from build123d import *

# Parameters (mm, degrees)
SKETCH_1_W          = 200
SKETCH_1_H          = 170
EXTRUDE_1_DEPTH     = 1
SKETCH_2_R          = 52.5
CUT_EXTRUDE_1_DEPTH = 2
SKETCH_3_R          = 1.6
CUT_EXTRUDE_2_DEPTH = 1
SKETCH_6_W          = 1.1
SKETCH_6_H          = 170
CUT_EXTRUDE_4_DEPTH = 10
FILLET_1_R          = 2
SKETCH_8_R          = 1.6
CUT_EXTRUDE_5_DEPTH = 10


with BuildPart() as part:
    # 草图1 → 凸台-拉伸1 (new body)
    with BuildSketch(Plane.XY):
        Rectangle(SKETCH_1_W, SKETCH_1_H)
    extrude(amount=EXTRUDE_1_DEPTH)

    # 草图2 → 切除-拉伸1 (cut)
    with BuildSketch(Plane(origin=(0, 0, 0), x_dir=(-1, 0, 0), z_dir=(0, 0, -1))):
        with Locations((0, -95)):
            Circle(SKETCH_2_R)
    extrude(amount=-CUT_EXTRUDE_1_DEPTH, mode=Mode.SUBTRACT)

    # 草图3 → 切除-拉伸2 (cut)
    with BuildSketch(Plane(origin=(0, 0, 0), x_dir=(-1, 0, 0), z_dir=(0, 0, -1))):
        with Locations((95, 14.722484501)):
            Circle(SKETCH_3_R)
        with Locations((95, -5.277515499)):
            Circle(SKETCH_3_R)
    cut_extrude_2 = extrude(amount=-CUT_EXTRUDE_2_DEPTH, mode=Mode.SUBTRACT)

    # 镜向1: 切除-拉伸2 across plane
    add(cut_extrude_2.mirror(Plane(origin=(0, 0, 0), x_dir=(0, 0, 1), z_dir=(1, 0, 0))), mode=Mode.SUBTRACT)

    # 草图6 → 切除-拉伸4 (cut)
    with BuildSketch(Plane(origin=(0, 0, 0), x_dir=(-1, 0, 0), z_dir=(0, 0, -1))):
        with Locations((-99.45, 0)):
            Rectangle(SKETCH_6_W, SKETCH_6_H)
    extrude(amount=-CUT_EXTRUDE_4_DEPTH, mode=Mode.SUBTRACT)

    # 圆角1
    fillet_1_edges = [part.edges().sort_by_distance(p)[0] for p in [
        (51.53882032, -85, 0.5),
        (-51.53882032, -85, 0.5),
        (98.9, 85, 0.5),
        (98.9, -85, 0.5),
        (-100, -85, 0.5),
        (-100, 85, 0.5),
    ]]
    fillet(fillet_1_edges, radius=FILLET_1_R)

    # 草图8 → 切除-拉伸5 (cut)
    with BuildSketch(Plane(origin=(0, 0, 0), x_dir=(-1, 0, 0), z_dir=(0, 0, -1))):
        with Locations((-92.1, 44.5)):
            Circle(SKETCH_8_R)
        with Locations((-92.1, 30.5)):
            Circle(SKETCH_8_R)
        with Locations((-92.1, -30.5)):
            Circle(SKETCH_8_R)
        with Locations((-92.1, -44.5)):
            Circle(SKETCH_8_R)
    extrude(amount=-CUT_EXTRUDE_5_DEPTH, mode=Mode.SUBTRACT)


solid = part.part
Source: CAD feature listing. Evaluate the final solid. Frame: model axes, mm. Round coordinates to 2 decimals unless told otherwise and drop trailing zeros. Loops run counter-clockwise (first coordinate to the right, second up) from the corner with the lowest first, then second, coordinate; pieces in that order, holes last. Notation, with made-up numbers: (-3, 7.25) - (38, 7.25) arc R11 cw to (38, 21.25) - close; hole circle Ø9 at (-4.5, 2.5). An arc over 180 degrees is marked (long way). Write item = value, one per line. Start each with the question number.
(1) Pull-direction query (X, two-part tool) for faces 1 (the face through (-2, 1, 0)), 2 (the face through (-0.99, -42.51, 0.49)); classes: +X half, -X half, draft (parallel to the pull), parting line (faces both ways), or undercut.
(2) Pin query (flat end, axial travel): pin 1 (1 mm diameter, centred on x = 76, y = -57.5, fed in from -Z). Return the tip coordinate at first contact, or that it passes through.
(3) Section query B-B, the plane z = 0.45. State how many separate pieces and enclosed holes the cut face has, plus the area to 3 significant figures.
(4) Section query A-A, the plane y = -55.5. Output: boundary loops of the cut face in (x, z).
(5) Ray query, line 1 along Y through (x, z) = (95, 0.6); line 2 along Y through (x, z) = (92.1, 0.35); line 3 along Y through (x, z) = (21.5, 0.8). Return the intervals inside material, ascending. Write a range as from..to.
(6) Section query C-C, the plane x = 1. Output: boundary loops of the cut face in (y, z), plus the area to 3 significant figures.
(7) Section query D-D, the plane x = 40. Output: boundary loops of the cut face in (y, z), plus the area to 3 significant figures.
Conclusion:
q1.face_1 = draft
q1.face_2 = undercut
q2.pin_1 = 0
q3.separate_pieces = 1
q3.enclosed_holes = 8
q3.area = 30,500 mm2
q4.outline = (-100, 0) - (-34.58, 0) - (-34.58, 1) - (-100, 1) - close; (34.58, 0) - (98.9, 0) - (98.9, 1) - (34.58, 1) - close
q5.line_1 = -85..-6.88, -3.68..13.12, 16.32..85
q5.line_2 = -85..-46.1, -42.9..-32.1, -28.9..28.9, 32.1..42.9, 46.1..85
q5.line_3 = -47.1..85
q6.outline = (-42.51, 0) - (85, 0) - (85, 1) - (-42.51, 1) - close
q6.area = 128 mm2
q7.outline = (-61, 0) - (85, 0) - (85, 1) - (-61, 1) - close
q7.area = 146 mm2
